Could you check a few things on this model? Use its own coordinates, in mm. Face numbers are marked on the shaded views. A direction names the side the tool comes from. Round coordinates to 2 decimals unless told otherwise and drop trailing zeros. Order: outer loops, then holes, each group sorted by start corner. A loop starts at its lowest first (then second) coordinate and runs counter-clockwise, first axis right, second up.
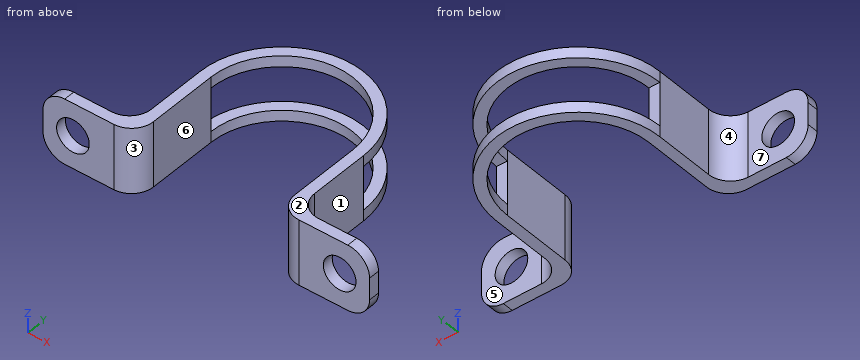
```python
from build123d import *

# Parameters (mm, degrees)
BOSS_EXTRUDE1_DEPTH     = 6
SKETCH2_R               = 1.5
CUT_EXTRUDE1_DEPTH      = 6
CUT_EXTRUDE2_DEPTH      = 12
CUT_EXTRUDE2_DEPTH_BACK = 17
SKETCH3_W               = 4
SKETCH3_H               = 10
FILLET1_R               = 2


with BuildPart() as part:
    # Sketch1 → Boss-Extrude1 (new body)
    with BuildSketch(Plane.XY):
        with BuildLine():
            Line((-15, 0), (-9.5, 0))
            ThreePointArc((-9.5, 0), (-8.085786438, 0.585786438), (-7.5, 2))
            Line((-7.5, 2), (-7.5, 7.5))
            ThreePointArc((-7.5, 7.5), (0, 15), (7.5, 7.5))
            Line((7.5, 7.5), (7.5, 2))
            ThreePointArc((7.5, 2), (8.085786438, 0.585786438), (9.5, 0))
            Line((9.5, 0), (15, 0))
            Line((15, 0), (15, -1))
            Line((15, -1), (8.5, -1))
            ThreePointArc((8.5, -1), (7.085786438, -0.414213562), (6.5, 1))
            Line((6.5, 1), (6.5, 7.5))
            ThreePointArc((6.5, 7.5), (0, 14), (-6.5, 7.5))
            Line((-6.5, 7.5), (-6.5, 1))
            ThreePointArc((-6.5, 1), (-7.085786438, -0.414213562), (-8.5, -1))
            Line((-8.5, -1), (-15, -1))
            Line((-15, -1), (-15, 0))
        make_face()
    extrude(amount=BOSS_EXTRUDE1_DEPTH)

    # Sketch2 → Cut-Extrude1 (cut)
    with BuildSketch(Plane(origin=(0, 0, 0), x_dir=(1, 0, 0), z_dir=(0, 1, 0))):
        with Locations(Location((12.25, -3, 0), (0, 0, 270))):
            Circle(SKETCH2_R)
        with Locations(Location((-12.25, -3, 0), (0, 0, 180))):
            Circle(SKETCH2_R)
    extrude(amount=-CUT_EXTRUDE1_DEPTH, mode=Mode.SUBTRACT)

    # Sketch3 → Cut-Extrude2 (cut, two sides: drawn at the far end of the back side and taken through both)
    with BuildSketch(Plane(origin=(0, 0, 0), x_dir=(0, 0, -1), z_dir=(1, 0, 0)).offset(-CUT_EXTRUDE2_DEPTH_BACK)):
        with Locations((-3, 12.5)):
            Rectangle(SKETCH3_W, SKETCH3_H)
    extrude(amount=CUT_EXTRUDE2_DEPTH + CUT_EXTRUDE2_DEPTH_BACK, mode=Mode.SUBTRACT)

    # Fillet1
    fillet1_edges = [part.edges().sort_by_distance(p)[0] for p in [
        (15, -0.5, 0),
        (-15, -0.5, 0),
        (15, -0.5, 6),
        (-15, -0.5, 6),
    ]]
    fillet(fillet1_edges, radius=FILLET1_R)


solid = part.part
```
Q1. Imagine slicing it at D-D, the plane z = 5.35. Please give me the cut outline in (x, y).
Q2. For the marked faces 5, 6 and 7, which set-ups out of +Z, -Z, +X, -X, +Y, -Y let a thin tool reach every point of the face, with its end or its side?
Q3. Imagine slicing it at C-C, the plane y = 8. Please give me the cut outline in (x, z).
Q4. Imagine slicing it at A-A, the plane x = -12.25. Please give me the cut outline in (y, z), then the cut area to 3 significant figures.
Q5. For P1, Ø1.1, axis at x = -7, z = 3, coming from the +Y side; P2, Ø6, axis at x = -1.5, y = 12, coming from the +Z side; P3, Ø2, axis at x = 1.5, z = 0.5, coming from the +Y side; P4, Ø1.6, axis at x = -11.5, z = 4, coming from the +Y side, each with a flat end and sliding along its axis, tell me the tip position at first contact or that it passes through.
Q6. I need wall thicknesses on L1, parallel to X at y = 6.5, z = 5.05; L2, parallel to Z at x = -12.25, y = -0.3; L3, parallel to Z at x = 7, y = 8. Which ranges of each line are inside material? Lowest first, please.
Q7. We'd pull the mould along X, two halves only. Please class the marked faces 1, 2, 3 and 4: released by +X, released by -X, zero draft, split by the parting line, or undercut.
Q8. Imagine slicing it at B-B, the plane y = 3. Please give me the cut outline in (x, z).
Filled in:
1. outline: (-14.48, -1) - (-8.5, -1) arc R2 ccw to (-6.5, 1) - (-6.5, 7.5) arc R6.5 cw to (6.5, 7.5) - (6.5, 1) arc R2 ccw to (8.5, -1) - (14.48, -1) - (14.48, 0) - (9.5, 0) arc R2 cw to (7.5, 2) - (7.5, 7.5) arc R7.5 ccw to (-7.5, 7.5) - (-7.5, 2) arc R2 cw to (-9.5, 0) - (-14.48, 0) - close
2. face 5: +Z, -Z, +X, +Y
2. face 6: +Z, -Z, -Y
2. face 7: +Z, -Z, -X, +Y
3. outline: (-7.48, 0) - (-6.48, 0) - (-6.48, 1) - (-7.48, 1) - close; (-7.48, 5) - (-6.48, 5) - (-6.48, 6) - (-7.48, 6) - close; (6.48, 0) - (7.48, 0) - (7.48, 1) - (6.48, 1) - close; (6.48, 5) - (7.48, 5) - (7.48, 6) - (6.48, 6) - close
4. outline: (-1, 0) - (0, 0) - (0, 1.5) - (-1, 1.5) - close; (-1, 4.5) - (0, 4.5) - (0, 6) - (-1, 6) - close
4. area: 3.00 mm2
5. P1: stops at y = 7.5
5. P2: stops at z = 6
5. P3: stops at y = 14.98
5. P4: stops at y = 0
6. L1: x = -7.5 to -6.5, 6.5 to 7.5
6. L2: z = 0 to 1.5, 4.5 to 6
6. L3: z = 0 to 1, 5 to 6
7. face 1: released by +X
7. face 2: zero draft
7. face 3: undercut
7. face 4: released by -X
8. outline: (-7.5, 0) - (-6.5, 0) - (-6.5, 6) - (-7.5, 6) - close; (6.5, 0) - (7.5, 0) - (7.5, 6) - (6.5, 6) - close
